```python
from build123d import *

# Parameters (mm, degrees)
BOSS_EXTRUDE1_DEPTH = 8
BOSS_EXTRUDE2_START = 1
SKETCH2_R           = 6
BOSS_EXTRUDE2_DEPTH = 1
CUT_EXTRUDE1_DEPTH  = 15.730919863
CUT_EXTRUDE2_DEPTH  = 2.9
HOLEWZD1_D          = 3.5
HOLEWZD1_DEPTH      = 3
FILLET1_R           = 0.6
FILLET2_R           = 2


with BuildPart() as part:
    # Sketch1 → Boss-Extrude1 (new body)
    with BuildSketch(Plane.XY.offset(-1)):
        with BuildLine():
            Line((8.660254038, 5), (1.820011325, 5.943700987))
            ThreePointArc((1.820011325, 5.943700987), (-5, 0), (1.820011325, -5.943700987))
            Line((1.820011325, -5.943700987), (8.660254038, -5))
            ThreePointArc((8.660254038, -5), (10, 0), (8.660254038, 5))
        make_face()
    extrude(amount=-BOSS_EXTRUDE1_DEPTH)

    # Sketch2 → Boss-Extrude2 (add)
    with BuildSketch(Plane.XY.offset(-1).offset(BOSS_EXTRUDE2_START)):
        with Locations((1, 0)):
            Circle(SKETCH2_R)
    extrude(amount=-BOSS_EXTRUDE2_DEPTH)

    # Sketch3 → Cut-Extrude1 (cut, through all)
    with BuildSketch(Plane.XY):
        with BuildLine():
            Line((0, -3.75), (4.1, -3.75))
            Line((4.1, -3.75), (4.1, 3.75))
            Line((4.1, 3.75), (0, 3.75))
            ThreePointArc((0, 3.75), (-3.75, 0), (0, -3.75))
        make_face()
    extrude(amount=-CUT_EXTRUDE1_DEPTH, mode=Mode.SUBTRACT)

    # Sketch4 → Cut-Extrude2 (cut)
    with BuildSketch(Plane.ZY.offset(-4.1)):
        Polygon((-9, -3), (-3.267949192, -3), (-1.535898385, 0), (-3.267949192, 3), (-9, 3), align=None)
    extrude(amount=-CUT_EXTRUDE2_DEPTH, mode=Mode.SUBTRACT)

    # HoleWzd1
    with Locations(Plane.ZY.offset(-7)):
        with Locations((-5, 0)):
            Hole(HOLEWZD1_D / 2, depth=HOLEWZD1_DEPTH)

    # Fillet1
    fillet1_edges = [part.edges().sort_by_distance(p)[0] for p in [
        (4.1, -3, -6.133974596),
        (4.1, 3, -6.133974596),
    ]]
    fillet(fillet1_edges, radius=FILLET1_R)

    # Fillet2
    fillet2_edges = [part.edges().sort_by_distance(p)[0] for p in [
        (8.660254038, -5, -5),
        (8.660254038, 5, -5),
    ]]
    fillet(fillet2_edges, radius=FILLET2_R)


solid = part.part
```
Input: part model. Units: mm. Frame: model coordinates. A direction names the side the tool comes from. Give positions to 0.01 mm unless a question says otherwise; leave off trailing zeros. Loops run counter-clockwise (first coordinate to the right, second up) from the corner with the lowest first, then second, coordinate; pieces in that order, holes last. Notation, with made-up numbers: M -22,-1 L 5,-1 A7 ccw 5,7 Z; hole C 28,-14.5 d8. An arc over 180 degrees is marked long. Answer as CSV lines item,"result". Start each with the question number.
1. Section B-B on y = 2.25. Return loops of the section in (x, z).
2. Pin query (flat end, axial travel): P1, Ø1.2, axis at x = 2.5, z = -4, coming from the -Y side; P2, Ø4, axis at x = 3.5, y = 1, coming from the -Z side; P3, Ø1, axis at x = -3.5, z = -3.5, coming from the +Y side. Return the tip coordinate at first contact, or that it passes through.
3. Pull-direction query (Y, two-part tool) for faces 6 (the face through (8, 0, -1)), 7 (the face through (-3.75, 0.08, -4.44)), 8 (the face through (4.68, -5.55, -4.94)); classes: released by +Y, released by -Y, zero draft, split by the parting line, or undercut.
4. Line query: L1, parallel to Z at x = 9.05, y = 0; L2, parallel to Z at x = 8.5, y = 4.5; L3, parallel to Y at x = 6, z = -5.25. Output: solid intervals per line, ascending.
5. Section D-D on y = 0.25. Return loops of the section in (x, z).
6. Section C-C on z = -5.75. Return loops of the section in (x, y), plus the area to 3 significant figures.
7. Section A-A on x = 1. Return loops of the section in (y, z), plus the area to 3 significant figures.
8. Reachability of faces 1 (the face through (8.572, 4.744, -5.056)), 2 (the face through (8.521, 0.526, -6.669)), 3 (the face through (2, -3.75, -4)), 4 (the face through (5, 0, 0)), 5 (the face through (6, -3, -6)) from +Z, -Z, +X, -X, +Y, -Y: full face, straight path, thin tool, end or side. Return the list, or none.
Computed values:
1,outline,"M -4.56,-9 L -3,-9 L -3,0 L -4.56,0 Z; M 4.1,-2.83 L 7,-2.83 L 7,-9 L 9.74,-9 L 9.74,-1 L 6.56,-1 L 6.56,0 L 4.1,0 Z"
2,P1,"stops at y = -5.93"
2,P2,"stops at z = -3.21"
2,P3,"stops at y = 4.47"
3,face 6,"zero draft"
3,face 7,"undercut"
3,face 8,"released by -Y"
4,L1,"z = -9 to -6.75, -3.25 to -1"
4,L2,"z = -9 to -1"
4,L3,"y = -5.37 to -3, 3 to 5.37"
5,outline,"M -4.99,-9 L -3.74,-9 L -3.74,0 L -4.99,0 Z; M 4.1,-1.68 L 7,-1.68 L 7,-3.27 L 10,-3.27 L 10,-1 L 6.99,-1 L 6.99,0 L 4.1,0 Z; M 7,-9 L 10,-9 L 10,-6.73 L 7,-6.73 Z"
6,outline,"M 0,-3.75 A3.75 cw 0,3.75 L 4.1,3.75 L 4.1,3.6 A0.6 ccw 4.7,3 L 7,3 L 7,1.58 L 9.87,1.58 A10 ccw 9.19,3.95 A2 ccw 7.62,5.14 L 1.82,5.94 A6 ccw long 1.82,-5.94 L 7.62,-5.14 A2 ccw 9.19,-3.95 A10 ccw 9.87,-1.58 L 7,-1.58 L 7,-3 L 4.7,-3 A0.6 ccw 4.1,-3.6 L 4.1,-3.75 Z"
6,area,"70.2 mm²"
7,outline,"M -6,-9 L -3.75,-9 L -3.75,0 L -6,0 Z; M 3.75,-9 L 6,-9 L 6,0 L 3.75,0 Z"
7,area,"40.5 mm²"
8,face 1,"+Z, -Z, +X, +Y"
8,face 2,"+X"
8,face 3,"+Z, -Z"
8,face 4,"+Z, +X, -X, +Y, -Y"
8,face 5,"-Z"
